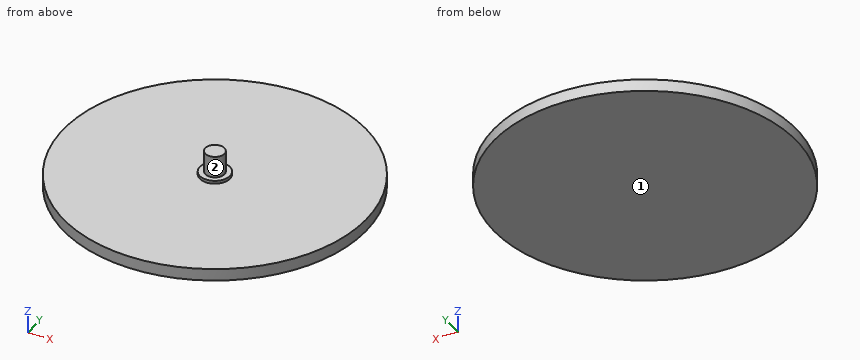
from build123d import *

# Parameters (mm, degrees)
F0_R       = 5
F0_R_2     = 3.175
F1_DEPTH   = 1
F2_R       = 3.175
F3_DEPTH   = 7.14
F0_R_3     = 50
F1_FACE1_R = 5
F4_DEPTH   = 4


with BuildPart() as f1:
    # F0 (on Top) → F1 (new body)
    with BuildSketch(Plane.XY):
        Circle(F0_R)
        Circle(F0_R_2, mode=Mode.SUBTRACT)
        Circle(F0_R_2)
    extrude(amount=F1_DEPTH)

    # F2 (on face) → F3 (join)
    with BuildSketch(Plane.XY.offset(1)):
        Circle(F2_R)
    extrude(amount=F3_DEPTH)

    # F0 (on Top) + F1_face1 (on face) → F4 (join)
    with BuildSketch(Plane.XY):
        Circle(F0_R_3)
        Circle(F0_R, mode=Mode.SUBTRACT)
    with BuildSketch(Plane(origin=(0, 0, 0), x_dir=(1, 0, 0), z_dir=(0, 0, -1))):
        Circle(F1_FACE1_R)
    extrude(amount=-F4_DEPTH, dir=(0, 0, 1))


solid = f1.part
Verification items for the finished model (mm, model axes). Face numbers are marked on the shaded views. A direction names the side the tool comes from. Coordinates: 2 decimals unless noted, no trailing zeros. Order: outer loops, then holes, each group sorted by start corner. A loop starts at its lowest first (then second) coordinate and runs counter-clockwise, first axis right, second up. Notation, with made-up numbers: M -13,-20.75 L -6,-20.75 A13 cw -6,-5.75 Z; hole C 0.25,59 d2. An arc over 180 degrees is marked long. Return JSON: item names as keys, results as strings.
1) Thickness scan on L1, parallel to Z at x = -5, y = 9.5; L2, parallel to X at y = 43.5, z = -3; L3, parallel to X at y = -8, z = -1.75. Record the ranges inside material, lowest first. Write a range as [from, to].
Answer list:
{"L1": "[-4, 0]", "L2": "[-24.65, 24.65]", "L3": "[-49.36, 49.36]"}
2) Gauge pin test, flat ends, axial feed: pin 1 (5 mm diameter, centred on x = -19, y = -29.5, fed in from +Z); pin 2 (1.5 mm diameter, centred on y = -22, z = 0, fed in from +X); pin 3 (1.5 mm diameter, centred on x = 9.5, z = 1, fed in from -Y); pin 4 (1.5 mm diameter, centred on y = 1, z = 3, fed in from -X). Record the tip position at first contact, or that the pin passes through.
Answer list:
{"pin 1": "z = 0", "pin 2": "x = 45.26", "pin 3": "through", "pin 4": "x = -3.17"}
3) Cross-section at C-C, the plane z = 2.25. Record the boundary of the cut face in (x, y) (3 decimals).
Answer list:
{"outline": "C 0,0 d6.35"}
4) Cross-section at A-A, the plane y = 0. Record the boundary of the cut face in (x, z) (3 decimals), and give its area (3 significant figures).
Answer list:
{"outline": "M -50,-4 L 50,-4 L 50,0 L 5,0 L 5,1 L 3.175,1 L 3.175,8.14 L -3.175,8.14 L -3.175,1 L -5,1 L -5,0 L -50,0 Z", "area": "455 mm2"}
5) Cross-section at D-D, the plane y = -23. Record the boundary of the cut face in (x, z), and give its area (3 significant figures).
Answer list:
{"outline": "M -44.4,-4 L 44.4,-4 L 44.4,0 L -44.4,0 Z", "area": "355 mm2"}
6) Access from +Z, -Z, +X, -X, +Y, -Y to the whole of each face (thin tool, end or side, straight path). Record for the marked faces 1 and 2.
Answer list:
{"face 1": "-Z, +X, -X, +Y, -Y", "face 2": "+Z"}
